Build history of the part. All positions in model axes, mm. A direction names the side the tool comes from. Give positions to 0.01 mm unless a question says otherwise; leave off trailing zeros. Write each loop counter-clockwise with the first axis right and the second up, starting at its lowest first coordinate (ties: lowest second). Pieces come first, ordered by that corner, then holes. Notation, with made-up numbers: M -38,-35 L 11,-35 A19 cw 11,-17 Z; hole C 27,13.5 d6. An arc over 180 degrees is marked long. Return JSON: item names as keys, results as strings. Group by question number.
Q1. Tool access for faces 5 (the cylindrical face through (-24.41, 8.11, 7.88)), 6 (the flat face through (-13, -6, -12.5)), 7 (the flat face through (-21, -6.5, 0)): list every direction of +Z, -Z, +X, -X, +Y, -Y with a clear straight run to the whole face (end or side of a thin tool).
Q2. Band-saw the part on D-D, the plane y = 2. Give the cut face in (x, z).
Q3. Band-saw the part on B-B, the plane x = -30. Give the cut face in (y, z), then the cut area to 3 significant figures.
Q4. Wall check: probe 1 along Y at (x, z) = (-31, -2.5); probe 2 along X at (y, z) = (-12, 12); probe 3 along Z at (x, y) = (-27, -2). Give the ranges that are in metal, low to high.
Q5. Flat gauge pins, fed straight in: pin 1 Ø1.5 at (x, z) = (-28, 16) entering from -Y; pin 2 Ø18 at (x, y) = (-9, -16) entering from +Z; pin 3 Ø2 at (x, y) = (-19.5, 2.5) entering from +Z; pin 4 Ø2 at (y, z) = (0, 3) entering from +X. Where does each tip first touch, or does it go through?
Q6. Band-saw the part on C-C, the plane z = -10.25. Give the cut face in (x, y), then the cut area to 3 significant figures.
Q7. Pull direction Y, two halves, no side cores. Call faces 1 (the flat face through (-26, 0, 14)), 2 (the flat face through (-26, 16, 12)), 3 (the cylindrical face through (-3.26, -9.63, -2.22)), 4 (the flat face through (-13, -6, 12.5)): +Y half, -Y half, draft (parallel to the pull), parting line (faces both ways), or undercut.
Q8. Band-saw the part on A-A, the plane z = -1.5. Give the cut face in (x, y).
from build123d import *

# Parameters (mm, degrees)
SALIENTE_EXTRUIR1_DEPTH = 12.5
CROQUIS5_R              = 2.5
CORTAR_EXTRUIR1_DEPTH   = 25
CROQUIS15_W             = 5
CROQUIS15_H             = 16


with BuildPart() as part:
    # Croquis1 → Saliente-Extruir1 (new, symmetric)
    with BuildSketch(Plane.XY):
        Polygon((-35.162289575, 0), (-0.162289575, 0), (0, -22.757556118), (-6.5, -22.757556118), (-6.5, -6.5), (-35.162289575, -6.5), align=None)
    extrude(amount=SALIENTE_EXTRUIR1_DEPTH, both=True)

    # Croquis5 → Cortar-Extruir1 (cut)
    with BuildSketch(Plane(origin=(-0.162281322, -0.001157267, 0), x_dir=(0, 0, -1), z_dir=(0.9999745736838829, 0.007131057827339795, 0))):
        with Locations(Location((0, -10.756977477, 0), (0, 0, 90))):
            Circle(CROQUIS5_R)
    extrude(amount=-CORTAR_EXTRUIR1_DEPTH, mode=Mode.SUBTRACT)

    # Croquis15 → Revolución2 (revolve)
    with BuildSketch(Plane.XY.offset(12.5), mode=Mode.PRIVATE) as revoluci_n2_sk:
        with Locations((-23.826251853, 8)):
            Rectangle(CROQUIS15_W, CROQUIS15_H)
    revolve(revoluci_n2_sk.sketch.rotate(Axis((-26.326251853, 0, 12.5), (0, 1, 0)), 90), axis=Axis((-26.326251853, 0, 12.5), (0, 1, 0)))


solid = part.part
From the geometry:
{
 "1": {"face 5": "+Y", "face 6": "-Z, +X, -X, +Y, -Y", "face 7": "+Z, -Z, -X, -Y"},
 "2": {"outline": "C -26.33,12.5 d10"},
 "3": {"outline": "M -6.5,-12.5 L 0,-12.5 L 0,9.11 L 16,9.11 L 16,15.89 L 0,15.89 L 0,12.5 L -6.5,12.5 Z", "area": "271 mm^2"},
 "4": {"probe 1": "y = -6.5 to 0", "probe 2": "x = -6.5 to -0.08", "probe 3": "z = -12.5 to 12.5"},
 "5": {"pin 1": "stops at y = 0", "pin 2": "stops at z = 12.5", "pin 3": "passes through", "pin 4": "stops at x = -0.16"},
 "6": {"outline": "M -35.16,-6.5 L -6.5,-6.5 L -6.5,-22.76 L 0,-22.76 L -0.16,0 L -35.16,0 Z", "area": "332 mm^2"},
 "7": {"face 1": "-Y half", "face 2": "+Y half", "face 3": "undercut", "face 4": "draft"},
 "8": {"outline": "M -35.16,-6.5 L -6.5,-6.5 L -6.5,-8.8 L -0.1,-8.76 L -0.16,0 L -35.16,0 Z; M -6.5,-22.76 L 0,-22.76 L -0.07,-12.76 L -6.5,-12.8 Z"}
}
